Here's how the part is built. I have some questions about the finished solid (model axes, mm). A direction names the side the tool comes from. Give positions to 0.01 mm unless a question says otherwise; leave off trailing zeros. Write each loop counter-clockwise with the first axis right and the second up, starting at its lowest first coordinate (ties: lowest second). Pieces come first, ordered by that corner, then holes. Notation, with made-up numbers: (7, -39) - (52, -39) arc R32 cw to (52, -1) - close; hole circle Ø7 at (-15.5, 31). An arc over 180 degrees is marked (long way). Write each question's results on one line, items separated by ' | '. Start each with the question number.
Item 1: Suppose I cut it at C-C on y = 25.4. List the corners of the cut face in (x, z) for me.
Item 2: Suppose I cut it at A-A on y = 0. List the corners of the cut face in (x, z) for me.
Item 3: Will these pins go through, and if not, where does the flat tip stop? P1, Ø2, axis at y = 0, z = 8.128, coming from the -X side; P2, Ø12, axis at x = 12, y = 13, coming from the -Z side; P3, Ø11, axis at x = 7, z = -19, coming from the -Y side; P4, Ø2, axis at y = 55.5, z = -25, coming from the +X side.
Item 4: Suppose I cut it at B-B on z = 0. List the corners of the cut face in (x, y) for me.
Item 5: Suppose I cut it at D-D on x = 52. List the corners of the cut face in (y, z) for me.
Item 6: Please list where these lines run through material, in increasing order: line 1 along Y through (x, z) = (7.5, 0); line 2 along Y through (x, z) = (115.25, 0); line 3 along Z through (x, y) = (111, 25).
Item 7: We'd pull the mould along Z, two halves only. Please class faces 5 (the cylindrical face through (4.884, -4.897, 1.087)), 6 (the flat face through (4.884, 60.747, -34.255)), 7 (the flat face through (107.3, 25, 0)), 8 (the flat face through (64, 31.446, 0)): +Z half, -Z half, draft (parallel to the pull), parting line (faces both ways), or undercut.
Item 8: Which directions (+Z, -Z, +X, -X, +Y, -Y) give clear straight access to the entire face, cutting with the end or side of a thin tool? Please do faces 1 (the flat face through (5, 56.973, 0)), 2 (the flat face through (46, 27, 6.35)), 3 (the flat face through (55, 27, -6.35)), 4 (the cylindrical face through (113.739, 30.437, 0.661)).
```python
from build123d import *

# Parameters (mm, degrees)
SKETCH1_R           = 5.0165
SKETCH1_R_2         = 1.778
BOSS_EXTRUDE1_DEPTH = 9.906
BOSS_EXTRUDE2_DEPTH = 9.906
BOSS_EXTRUDE3_START = -9.906
SKETCH4_W           = 12.7
SKETCH4_H           = 12.091045256
BOSS_EXTRUDE3_DEPTH = 110.094000005
SKETCH5_R           = 5.08
CUT_EXTRUDE1_DEPTH  = 12.7


with BuildPart() as part:
    # Sketch1 → Boss-Extrude1 (new body)
    with BuildSketch(Plane(origin=(0, 0, 0), x_dir=(0, 0, -1), z_dir=(1, 0, 0))):
        with BuildLine():
            Line((-6.35, 10.998522628), (-6.35, 51.892522628))
            Line((-6.35, 51.892522628), (6.35, 51.892522628))
            Line((6.35, 51.892522628), (6.35, 10.998522628))
            ThreePointArc((6.35, 10.998522628), (0, -12.7), (-6.35, 10.998522628))
        make_face()
        Circle(SKETCH1_R, mode=Mode.SUBTRACT)
        with Locations((-8.128, 0)):
            Circle(SKETCH1_R_2, mode=Mode.SUBTRACT)
        with Locations((0, 8.128)):
            Circle(SKETCH1_R_2, mode=Mode.SUBTRACT)
        with Locations((8.128, 0)):
            Circle(SKETCH1_R_2, mode=Mode.SUBTRACT)
        with Locations((0, -8.128)):
            Circle(SKETCH1_R_2, mode=Mode.SUBTRACT)
    extrude(amount=BOSS_EXTRUDE1_DEPTH)

    # Sketch3 → Boss-Extrude2 (add)
    with BuildSketch(Plane(origin=(0, 0, 0), x_dir=(0, 0, -1), z_dir=(1, 0, 0))):
        Polygon((-25.4, 51.892522628), (0, 51.892522628), (0, 56.972522628), (-23.295795103, 56.972522628), (-39.768409794, 73.445137319), (-43.360512242, 69.85303487), align=None)
        Polygon((0, 51.892522628), (25.4, 51.892522628), (43.360512242, 69.85303487), (39.768409794, 73.445137319), (23.295795103, 56.972522628), (0, 56.972522628), align=None)
    extrude(amount=BOSS_EXTRUDE2_DEPTH)

    # Sketch4 → Boss-Extrude3 (add)
    with BuildSketch(Plane.ZY.offset(BOSS_EXTRUDE3_START)):
        with Locations((0, 25.4)):
            Rectangle(SKETCH4_W, SKETCH4_H)
    extrude(amount=-BOSS_EXTRUDE3_DEPTH)

    # Sketch5 → Cut-Extrude1 (cut)
    with BuildSketch(Plane(origin=(120.000000005, 0, 0), x_dir=(0, 0, -1), z_dir=(1, 0, 0))):
        with Locations((0, 25.4)):
            Circle(SKETCH5_R)
    extrude(amount=-CUT_EXTRUDE1_DEPTH, mode=Mode.SUBTRACT)


solid = part.part
```
Checked values:
1) outline: (0, -6.35) - (120, -6.35) - (120, -5.08) - (107.3, -5.08) - (107.3, 5.08) - (120, 5.08) - (120, 6.35) - (0, 6.35) - close
2) outline: (0, -12.7) - (9.91, -12.7) - (9.91, -9.91) - (0, -9.91) - close; (0, -6.35) - (9.91, -6.35) - (9.91, -5.02) - (0, -5.02) - close; (0, 5.02) - (9.91, 5.02) - (9.91, 6.35) - (0, 6.35) - close; (0, 9.91) - (9.91, 9.91) - (9.91, 12.7) - (0, 12.7) - close
3) P1: passes through | P2: stops at z = -10.34 | P3: stops at y = 51.89 | P4: stops at x = 9.91
4) outline: (0, -12.7) - (9.91, -12.7) - (9.91, -9.91) - (0, -9.91) - close; (0, -6.35) - (9.91, -6.35) - (9.91, -5.02) - (0, -5.02) - close; (0, 5.02) - (9.91, 5.02) - (9.91, 6.35) - (0, 6.35) - close; (0, 9.91) - (9.91, 9.91) - (9.91, 19.35) - (120, 19.35) - (120, 20.32) - (107.3, 20.32) - (107.3, 30.48) - (120, 30.48) - (120, 31.45) - (9.91, 31.45) - (9.91, 56.97) - (0, 56.97) - close
5) outline: (19.35, -6.35) - (31.45, -6.35) - (31.45, 6.35) - (19.35, 6.35) - close
6) line 1: y = -12.7 to -9.91, -6.35 to -5.02, 5.02 to 6.35, 9.91 to 56.97 | line 2: y = 19.35 to 20.32, 30.48 to 31.45 | line 3: z = -6.35 to -5.06, 5.06 to 6.35
7) face 5: undercut | face 6: -Z half | face 7: undercut | face 8: draft
8) face 1: +X, -X, +Y | face 2: +Z, +X, -X | face 3: -Z, +X, -X | face 4: +X
